from build123d import *

# Parameters (mm, degrees)
SKETCH1_W                   = 406.4
SKETCH1_H                   = 457.2
BOSS_EXTRUDE1_DEPTH         = 3.175
CUT_EXTRUDE1_REACH          = 307.873
SKETCH2_W                   = 28.575
SKETCH2_H                   = 127
F_1_4_0_25_DIAMETER_HOLE1_D = 6.35


with BuildPart() as part:
    # Sketch1 → Boss-Extrude1 (new body)
    with BuildSketch(Plane(origin=(0, 0, 0), x_dir=(1, 0, 0), z_dir=(0, 1, 0))):
        Rectangle(SKETCH1_W, SKETCH1_H)
    extrude(amount=BOSS_EXTRUDE1_DEPTH)

    # Sketch2 → Cut-Extrude1 (cut, up to next)
    with BuildSketch(Plane(origin=(0, 3.175, 0), x_dir=(1, 0, 0), z_dir=(0, 1, 0)), mode=Mode.PRIVATE) as cut_extrude1_sk1:
        with Locations((-188.9125, 165.1)):
            Rectangle(SKETCH2_W, SKETCH2_H)
    cut_extrude1_tool1 = extrude(cut_extrude1_sk1.sketch, amount=-CUT_EXTRUDE1_REACH, mode=Mode.PRIVATE) & part.part
    # Sketch2 → Cut-Extrude1 (cut, up to next)
    with BuildSketch(Plane(origin=(0, 3.175, 0), x_dir=(1, 0, 0), z_dir=(0, 1, 0)), mode=Mode.PRIVATE) as cut_extrude1_sk2:
        with Locations((188.9125, -165.1)):
            Rectangle(SKETCH2_W, SKETCH2_H)
    cut_extrude1_tool2 = extrude(cut_extrude1_sk2.sketch, amount=-CUT_EXTRUDE1_REACH, mode=Mode.PRIVATE) & part.part
    add(cut_extrude1_tool1.solids().sort_by_distance((-188.9125, 3.175, -165.1))[0], mode=Mode.SUBTRACT)
    add(cut_extrude1_tool2.solids().sort_by_distance((188.9125, 3.175, 165.1))[0], mode=Mode.SUBTRACT)

    # 1/4 (0.25) Diameter Hole1 (through all)
    with Locations(Plane(origin=(0, 3.175, 0), x_dir=(1, 0, 0), z_dir=(0, 1, 0))):
        with Locations((-190.5, -215.9), (190.5, 215.9), (0, 215.9), (0, -215.9)):
            Hole(F_1_4_0_25_DIAMETER_HOLE1_D / 2)


solid = part.part
CAD build for the part. Positions are in the model's coordinates, mm. Round coordinates to 2 decimals unless told otherwise and drop trailing zeros. Order: outer loops, then holes, each group sorted by start corner. A loop starts at its lowest first (then second) coordinate and runs counter-clockwise, first axis right, second up. Notation, with made-up numbers: (21, 6) -> (77, 6) arc R29 cw to (77, 29) -> close; hole circle Ø6 at (82.25, -2.5). An arc over 180 degrees is marked (long way). Write item = value, one per line. Start each with the question number.
(1) Cut at B-B, the plane z = 135. List the corners of the cut face in (x, y) (3 decimals), then the cut area to 3 significant figures.
(2) Cut at A-A, the plane y = 1.85. List the corners of the cut face in (x, z) (3 decimals), then the cut area to 3 significant figures.
(3) Probe line 1 (X direction, y = 1.8, z = -215.9) (3 decimals); line 2 (Z direction, x = 0, y = 1.9) (3 decimals); line 3 (Z direction, x = -190.5, y = 2.55) (3 decimals). List the from-to ranges inside material, lowest first. Write a range as [from, to].
(4) Pin check, flat tips, straight feed: P1, Ø1, axis at x = -189.5, y = 1, coming from the -Z side; P2, Ø1, axis at y = 1.5, z = 159, coming from the +X side (3 decimals); P3, Ø1, axis at y = 2, z = -145, coming from the -X side (3 decimals). Stop position of each tip, or through.
Model answer:
q1.outline = (-203.2, 0) -> (174.625, 0) -> (174.625, 3.175) -> (-203.2, 3.175) -> close
q1.area = 1,200 mm2
q2.outline = (-203.2, -101.6) -> (-174.625, -101.6) -> (-174.625, -228.6) -> (203.2, -228.6) -> (203.2, 101.6) -> (174.625, 101.6) -> (174.625, 228.6) -> (-203.2, 228.6) -> close; hole circle Ø6.35 at (-190.5, 215.9); hole circle Ø6.35 at (0, -215.9); hole circle Ø6.35 at (0, 215.9); hole circle Ø6.35 at (190.5, -215.9)
q2.area = 178,000 mm2
q3.line_1 = [-174.625, -3.175], [3.175, 187.325], [193.675, 203.2]
q3.line_2 = [-228.6, -219.075], [-212.725, 212.725], [219.075, 228.6]
q3.line_3 = [-101.6, 212.725], [219.075, 228.6]
q4.P1 = -101.6
q4.P2 = 174.625
q4.P3 = -174.625
